```python
from build123d import *

# Parameters (mm, degrees)
SM_BASE_FLANGE_1_DEPTH = 394
SKETCH_6_W             = 35
SKETCH_6_H             = 60
CUT_EXTRUDE_1_DEPTH    = 24
CUT_EXTRUDE_START      = -22
SKETCH_11_W            = 4
SKETCH_11_H            = 31.5
CUT_EXTRUDE_6_DEPTH    = 22
SKETCH_8_R             = 9
SKETCH_8_R_2           = 4
SKETCH_8_R_3           = 3.5
CUT_EXTRUDE_3_DEPTH    = 10
SKETCH_12_R            = 2.5
CUT_EXTRUDE_7_DEPTH    = 10
SKETCH_13_R            = 5.25
CUT_EXTRUDE_8_DEPTH    = 10
SKETCH_14_R            = 4.5
CUT_EXTRUDE_9_DEPTH    = 10
SKETCH_15_R            = 3.5
CUT_EXTRUDE_2621_DEPTH = 10


# Sheet-metal steps are written as plain solids
with BuildPart() as part:
    # Sketch 1 → Базовая кромка1 (new, symmetric)
    with BuildSketch(Plane.XY):
        with BuildLine():
            Line((0, 0), (0, -18))
            ThreePointArc((0, -18), (-1.171572875, -20.828427125), (-4, -22))
            Line((-4, -22), (-31, -22))
            ThreePointArc((-31, -22), (-32.414213562, -22.585786438), (-33, -24))
            Line((-33, -24), (-33, -116))
            ThreePointArc((-33, -116), (-32.414213562, -117.414213562), (-31, -118))
            Line((-31, -118), (0, -118))
            Line((0, -118), (0, -120))
            Line((0, -120), (-31, -120))
            ThreePointArc((-31, -120), (-33.828427125, -118.828427125), (-35, -116))
            Line((-35, -116), (-35, -24))
            ThreePointArc((-35, -24), (-33.828427125, -21.171572875), (-31, -20))
            Line((-31, -20), (-4, -20))
            ThreePointArc((-4, -20), (-2.585786438, -19.414213562), (-2, -18))
            Line((-2, -18), (-2, 0))
            Line((-2, 0), (0, 0))
        make_face()
    extrude(amount=SM_BASE_FLANGE_1_DEPTH, both=True)

    # Эскиз6 → Вырез-Вытянуть1 (cut)
    with BuildSketch(Plane(origin=(0, 0, 0), x_dir=(1, 0, 0), z_dir=(0, 1, 0))):
        with Locations((-17.5, -364)):
            Rectangle(SKETCH_6_W, SKETCH_6_H)
        with Locations((-17.5, 364)):
            Rectangle(SKETCH_6_W, SKETCH_6_H)
    extrude(amount=-CUT_EXTRUDE_1_DEPTH, mode=Mode.SUBTRACT)

    # Эскиз11 → Вырез-Вытянуть6 (cut)
    with BuildSketch(Plane(origin=(0, 0, 0), x_dir=(1, 0, 0), z_dir=(0, 1, 0)).offset(CUT_EXTRUDE_START)):
        with Locations((-2, 318.25)):
            Rectangle(SKETCH_11_W, SKETCH_11_H)
        with Locations((-2, -318.25)):
            Rectangle(SKETCH_11_W, SKETCH_11_H)
    extrude(amount=CUT_EXTRUDE_6_DEPTH, mode=Mode.SUBTRACT)

    # Эскиз8 → Вырез-Вытянуть3 (cut)
    with BuildSketch(Plane.ZY.offset(35)):
        with Locations(Location((-365, -70, 0), (0, 0, 270))):
            Circle(SKETCH_8_R)
        with Locations(Location((-325, -70, 0), (0, 0, 270))):
            Circle(SKETCH_8_R)
        with Locations(Location((-365, -50, 0), (0, 0, 270))):
            Circle(SKETCH_8_R_2)
        with Locations(Location((-365, -100, 0), (0, 0, 270))):
            Circle(SKETCH_8_R_2)
        with Locations(Location((-285, -50, 0), (0, 0, 270))):
            Circle(SKETCH_8_R_3)
        with Locations(Location((-285, -100, 0), (0, 0, 270))):
            Circle(SKETCH_8_R_3)
        with Locations(Location((285, -100, 0), (0, 0, 90))):
            Circle(SKETCH_8_R_3)
        with Locations(Location((285, -50, 0), (0, 0, 90))):
            Circle(SKETCH_8_R_3)
        with Locations(Location((365, -100, 0), (0, 0, 90))):
            Circle(SKETCH_8_R_2)
        with Locations(Location((365, -50, 0), (0, 0, 90))):
            Circle(SKETCH_8_R_2)
        with Locations(Location((325, -70, 0), (0, 0, 90))):
            Circle(SKETCH_8_R)
        with Locations(Location((365, -70, 0), (0, 0, 90))):
            Circle(SKETCH_8_R)
    extrude(amount=-CUT_EXTRUDE_3_DEPTH, mode=Mode.SUBTRACT)

    # Эскиз12 → Вырез-Вытянуть7 (cut)
    with BuildSketch(Plane.ZY.offset(2)):
        with Locations(Location((-292.5, -7, 0), (0, 0, 270))):
            Circle(SKETCH_12_R)
        with Locations(Location((-265.5, -7, 0), (0, 0, 270))):
            Circle(SKETCH_12_R)
        with Locations(Location((265.5, -7, 0), (0, 0, 90))):
            Circle(SKETCH_12_R)
        with Locations(Location((292.5, -7, 0), (0, 0, 90))):
            Circle(SKETCH_12_R)
    extrude(amount=-CUT_EXTRUDE_7_DEPTH, mode=Mode.SUBTRACT)

    # Эскиз13 → Вырез-Вытянуть8 (cut)
    with BuildSketch(Plane(origin=(0, -20, 0), x_dir=(1, 0, 0), z_dir=(0, 1, 0))):
        with Locations(Location((-14, 299, 0), (0, 0, 180))):
            Circle(SKETCH_13_R)
        with Locations((-14, -299)):
            Circle(SKETCH_13_R)
    extrude(amount=-CUT_EXTRUDE_8_DEPTH, mode=Mode.SUBTRACT)

    # Эскиз14 → Вырез-Вытянуть9 (cut)
    with BuildSketch(Plane(origin=(0, -118, 0), x_dir=(1, 0, 0), z_dir=(0, 1, 0))):
        with Locations(Location((-15, 230, 0), (0, 0, 180))):
            Circle(SKETCH_14_R)
        with Locations((-15, -230)):
            Circle(SKETCH_14_R)
        with Locations(Location((-15, 200, 0), (0, 0, 180))):
            Circle(SKETCH_14_R)
        with Locations((-15, -200)):
            Circle(SKETCH_14_R)
    extrude(amount=-CUT_EXTRUDE_9_DEPTH, mode=Mode.SUBTRACT)

    # Эскиз15 → Cut-Extrude 2621 (cut)
    with BuildSketch(Plane(origin=(0, 0, 0), x_dir=(0, 0, -1), z_dir=(1, 0, 0))):
        with Locations(Location((-200, -7, 0), (0, 0, 90))):
            Circle(SKETCH_15_R)
        with Locations(Location((200, -7, 0), (0, 0, 270))):
            Circle(SKETCH_15_R)
    extrude(amount=-CUT_EXTRUDE_2621_DEPTH, mode=Mode.SUBTRACT)


solid = part.part
```
The model under review builds one solid part; all positions refer to its coordinate system, in mm. A direction names the side the tool comes from. Give positions to 0.01 mm unless a question says otherwise; leave off trailing zeros. Write each loop counter-clockwise with the first axis right and the second up, starting at its lowest first coordinate (ties: lowest second). Pieces come first, ordered by that corner, then holes.
(1) Tool access review of faces 1 (the flat face through (-2, -9, 4)), 2 (the flat face through (-17, -22, 5)), 3 (the flat face through (-34, -75, -394)): name each direction out of +Z, -Z, +X, -X, +Y, -Y from which nothing blocks a thin tool from reaching the whole face with its end or side.
(2) Consider section C-C, the plane y = -87.5. Give the boundary of the cut face in (x, z), and give its area (3 significant figures).
(3) Consider section A-A, the plane z = -325. Give the boundary of the cut face in (x, y), and give its area (3 significant figures).
(4) Consider section B-B, the plane z = 54. Give the boundary of the cut face in (x, y), and give its area (3 significant figures).
(5) To check wall thickness, follow L1, parallel to Z at x = -34.2, y = -100; L2, parallel to Y at x = -21, z = -215.5; L3, parallel to Z at x = -15, y = -119.45. State the ranges of each line that lie inside material, in increasing order.
(6) For P1, Ø8, axis at y = -101, z = -226, coming from the +X side; P2, Ø2, axis at x = -33.5, z = -365, coming from the +Y side; P3, Ø4.5, axis at x = -26.5, y = -21.5, coming from the -Z side, all flat-tipped, find the tip position at first contact; note any pin that passes through.
(7) The part is to be moulded in two halves that separate along Y. For faces 4 (the cylindrical face through (-34.014, -71.951, 333.786)), 5 (the flat face through (-16, -118, 6)), 6 (the flat face through (-35, -71, 6)), 7 (the flat face through (-18, -20, 5)), say which applies: released by +Y, released by -Y, zero draft, split by the parting line, or undercut.
Returned:
1. face 1: +Z, -Z, -X, +Y
1. face 2: +Z, -Z, +X
1. face 3: -Z, +X, -X, +Y, -Y
2. outline: (-35, -394) - (-33, -394) - (-33, 394) - (-35, 394) - close
2. area: 1,580 mm2
3. outline: (-35, -116) arc R4 ccw to (-31, -120) - (0, -120) - (0, -118) - (-31, -118) arc R2 cw to (-33, -116) - (-33, -79) - (-35, -79) - close; (-35, -61) - (-33, -61) - (-33, -24) arc R2 cw to (-31, -22) - (-4, -22) - (-4, -20) - (-31, -20) arc R4 ccw to (-35, -24) - close
3. area: 283 mm2
4. outline: (-35, -116) arc R4 ccw to (-31, -120) - (0, -120) - (0, -118) - (-31, -118) arc R2 cw to (-33, -116) - (-33, -24) arc R2 cw to (-31, -22) - (-4, -22) arc R4 ccw to (0, -18) - (0, 0) - (-2, 0) - (-2, -18) arc R2 cw to (-4, -20) - (-31, -20) arc R4 ccw to (-35, -24) - close
4. area: 364 mm2
5. L1: z = -394 to -369, -361 to -288.5, -281.5 to 281.5, 288.5 to 361, 369 to 394
5. L2: y = -120 to -118, -22 to -20
5. L3: z = -394 to -234.5, -225.5 to -204.5, -195.5 to 195.5, 204.5 to 225.5, 234.5 to 394
6. P1: stops at x = -33
6. P2: stops at y = -24
6. P3: stops at z = -334
7. face 4: undercut
7. face 5: undercut
7. face 6: zero draft
7. face 7: released by +Y
